from build123d import *

# Parameters (mm, degrees)
BOSS_EXTRUDE1_DEPTH = 9
CHAMFER1_SIZE       = 2.5
CHAMFER1_SIZE2      = 4.330127019
FILLET1_R           = 3
SKETCH11_R          = 1.195625
SKETCH11_R_2        = 1.5
CUT_EXTRUDE1_DEPTH  = 6
CUT_EXTRUDE2_DEPTH  = 0.5


with BuildPart() as part:
    # Sketch4 → Boss-Extrude1 (new body)
    with BuildSketch(Plane.XY):
        with BuildLine():
            Line((0, 19.5), (0, 14.5))
            Line((0, 14.5), (4.250076152, 14.5))
            ThreePointArc((4.250076152, 14.5), (4.606701377, 14.350454632), (4.75, 13.991273797))
            Line((4.75, 13.991273797), (4.610359481, 5.991273797))
            ThreePointArc((4.610359481, 5.991273797), (4.460890265, 5.643374775), (4.110435633, 5.5))
            Line((4.110435633, 5.5), (0, 5.5))
            Line((0, 5.5), (0, 0))
            Line((0, 0), (5, 0))
            Line((5, 0), (5, 19.5))
            Line((5, 19.5), (0, 19.5))
        make_face()
    extrude(amount=BOSS_EXTRUDE1_DEPTH)

    # Chamfer1
    chamfer1_edges = [part.edges().sort_by_distance(p)[0] for p in [
        (0, 17, 9),
    ]]
    chamfer1_side = [part.faces().sort_by_distance(p)[0] for p in [
        (0.201308221, 17, 9),
    ]]
    chamfer(chamfer1_edges, length=CHAMFER1_SIZE, length2=CHAMFER1_SIZE2, reference=chamfer1_side[0])

    # Fillet1
    fillet1_edges = [part.edges().sort_by_distance(p)[0] for p in [
        (0, 17, 4.669872981),
    ]]
    fillet(fillet1_edges, radius=FILLET1_R)

    # Mirror1: part across plane


with BuildPart() as part_1:
    add(part.part)
    add(part.part.mirror(Plane(origin=(4.250076152, 14, 0), x_dir=(1, 0, 0), z_dir=(0, 0, -1))))

    # Sketch11 → Cut-Extrude1 (cut, through all)
    with BuildSketch(Plane(origin=(5, 0, 0), x_dir=(0, 0, -1), z_dir=(1, 0, 0))):
        with Locations((-5.5, 3)):
            Circle(SKETCH11_R)
        with Locations((0, 3)):
            Circle(SKETCH11_R_2)
        with BuildLine():
            Line((5, 4.195625), (6, 4.195625))
            ThreePointArc((6, 4.195625), (7.195625, 3), (6, 1.804375))
            Line((6, 1.804375), (5, 1.804375))
            ThreePointArc((5, 1.804375), (3.804375, 3), (5, 4.195625))
        make_face()
    extrude(amount=-CUT_EXTRUDE1_DEPTH, mode=Mode.SUBTRACT)

    # Sketch12 → Cut-Extrude2 (cut)
    with BuildSketch(Plane(origin=(0, 19.5, 0), x_dir=(1, 0, 0), z_dir=(0, 1, 0))):
        with BuildLine():
            Line((0, 3.866025404), (0, -3.866025404))
            ThreePointArc((0, -3.866025404), (0.102222521, -4.642482539), (0.401923789, -5.366025404))
            Line((0.401923789, -5.366025404), (2.5, -9))
            Line((2.5, -9), (5, -9))
            Line((5, -9), (5, 9))
            Line((5, 9), (2.5, 9))
            Line((2.5, 9), (0.401923789, 5.366025404))
            ThreePointArc((0.401923789, 5.366025404), (0.102222521, 4.642482539), (0, 3.866025404))
        make_face()
    extrude(amount=-CUT_EXTRUDE2_DEPTH, mode=Mode.SUBTRACT)


solid = part_1.part
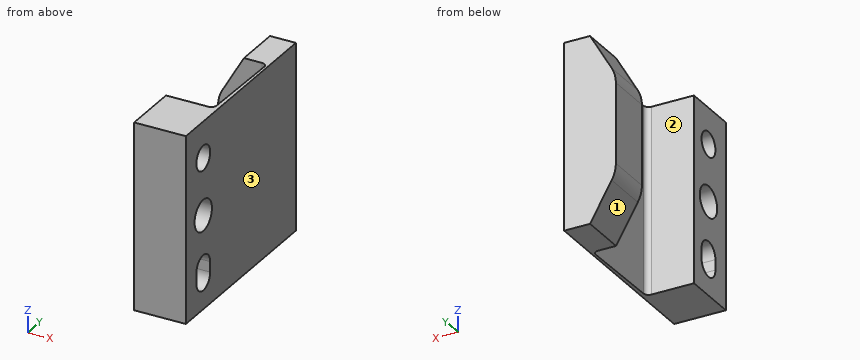
The model under review builds one solid part; all positions refer to its coordinate system, in mm. Face numbers are marked on the shaded views. A direction names the side the tool comes from. Give positions to 0.01 mm unless a question says otherwise; leave off trailing zeros. Loops run counter-clockwise (first coordinate to the right, second up) from the corner with the lowest first, then second, coordinate; pieces in that order, holes last. Notation, with made-up numbers: (-5.5, 45.25) -> (46.5, 45.25) arc R12 cw to (46.5, 64.25) -> close; hole circle Ø4 at (-22, 9.5). An arc over 180 degrees is marked (long way). Write each question's results on one line, items separated by ' | '.
1) Insertion check: pin 1 Ø2 at (x, z) = (2, -4.5) entering from -Y. The pin has a flat end and moves straight along its axis. Give the tip position at first contact, or say it passes through.
Conclusion:
pin 1: stops at y = 0
2) Tool access review of the marked faces 1, 2 and 3: name each direction out of +Z, -Z, +X, -X, +Y, -Y from which nothing blocks a thin tool from reaching the whole face with its end or side.
Conclusion:
face 1: -Z, -X, +Y | face 2: +Z, -Z, -X | face 3: +Z, -Z, +X, +Y, -Y
3) Take a section at C-C, the plane z = 0. Give the boundary of the cut face in (x, y), plus the area to 3 significant figures.
Conclusion:
outline: (0, 0) -> (5, 0) -> (5, 1.5) -> (0, 1.5) -> close; (0, 4.5) -> (5, 4.5) -> (5, 19) -> (0, 19) -> (0, 14.5) -> (4.25, 14.5) arc R0.5 cw to (4.75, 13.99) -> (4.61, 5.99) arc R0.5 cw to (4.11, 5.5) -> (0, 5.5) -> close | area: 38.0 mm^2
4) Take a section at D-D, the plane x = 2.2. Give the boundary of the cut face in (y, z), plus the area to 3 significant figures.
Conclusion:
outline: (0, -9) -> (5.5, -9) -> (5.5, 9) -> (0, 9) -> close; (14.5, -8.48) -> (19, -8.48) -> (19, 8.48) -> (14.5, 8.48) -> close; hole circle Ø3 at (3, 0); hole (1.8, -6) arc R1.2 ccw to (4.2, -6) -> (4.2, -5) arc R1.2 ccw to (1.8, -5) -> close; hole circle Ø2.39 at (3, 5.5) | area: 157 mm^2
5) Take a section at B-B, the plane y = 3. Give the boundary of the cut face in (x, z).
Conclusion:
outline: (0, -9) -> (5, -9) -> (5, -7.2) -> (0, -7.2) -> close; (0, -3.8) -> (5, -3.8) -> (5, -1.5) -> (0, -1.5) -> close; (0, 1.5) -> (5, 1.5) -> (5, 4.3) -> (0, 4.3) -> close; (0, 6.7) -> (5, 6.7) -> (5, 9) -> (0, 9) -> close
6) Take a section at A-A, the plane x = 3.75. Give the boundary of the cut face in (y, z), plus the area to 3 significant figures.
Conclusion:
outline: (0, -9) -> (5.5, -9) -> (5.5, 9) -> (0, 9) -> close; (14.5, -9) -> (19, -9) -> (19, 9) -> (14.5, 9) -> close; hole circle Ø3 at (3, 0); hole (1.8, -6) arc R1.2 ccw to (4.2, -6) -> (4.2, -5) arc R1.2 ccw to (1.8, -5) -> close; hole circle Ø2.39 at (3, 5.5) | area: 162 mm^2
7) For line 1 along Y through (x, z) = (3.35, 0); line 2 along Y through (x, z) = (3.2, 5.5); line 3 along Y through (x, z) = (2.9, 2.5), list the stretches that pass through material, from the lowest coordinate up. Write a range as from..to.
Conclusion:
line 1: y = 0..1.5, 4.5..5.5, 14.5..19 | line 2: y = 0..1.8, 4.2..5.5, 14.5..19 | line 3: y = 0..5.5, 14.5..19
